Check sheet for the modelled part. Datum: model origin and axes. Units: mm. A direction names the side the tool comes from. Give positions to 0.01 mm unless a question says otherwise; leave off trailing zeros. Write each loop counter-clockwise with the first axis right and the second up, starting at its lowest first coordinate (ties: lowest second). Pieces come first, ordered by that corner, then holes. Notation, with made-up numbers: M 66,-14.5 L 78,-14.5 A20 ccw 78,-6.5 Z; hole C 55,-11.5 d11. An arc over 180 degrees is marked long. Write each question's results on one line, items separated by ' | '. Start each with the question number.
from build123d import *

# Parameters (mm, degrees)
EXTRUDE_1_DEPTH      = 3
CUT_EXTRUDE_2_DEPTH  = 10
CUT_EXTRUDE_6_DEPTH  = 4
SKETCH_12_W          = 293.771267283
SKETCH_12_H          = 20
EXTRUDE_2_DEPTH      = 3
SKETCH_13_R          = 2
CUT_EXTRUDE_9_DEPTH  = 4
CUT_EXTRUDE_10_DEPTH = 10
MM_2_D               = 1.5
CUT_EXTRUDE_11_DEPTH = 4
MM_3_D               = 1.5
FILLET_1_R           = 2
EXTRUDE_3_DEPTH      = 3
SKETCH_4_R           = 1.5
CUT_EXTRUDE_3_DEPTH  = 10


with BuildPart() as part:
    # 草图1 → 凸台-拉伸1 (new body)
    with BuildSketch(Plane.XY):
        Polygon((-31.770103996, 71.767703031), (318.229896004, 71.767703031), (292.931935015, -47.249845949), (-31.770103996, 21.767703031), align=None)
    extrude(amount=EXTRUDE_1_DEPTH)

    # 草图3 → 切除-拉伸2 (cut)
    with BuildSketch(Plane.XY.offset(3)):
        Polygon((-0.469380772, 15.114528924), (0.1543543, 18.048971727), (-31.770103996, 24.834724815), (-31.770103996, 21.767703031), align=None)
        Polygon((176.220922432, -19.375132621), (205.565350454, -25.612483345), (204.941615382, -28.546926147), (175.59718736, -22.309575423), align=None)
    extrude(amount=-CUT_EXTRUDE_2_DEPTH, mode=Mode.SUBTRACT)

    # 草图7 → 切除-拉伸6 (cut, through all)
    with BuildSketch(Plane.XY.offset(3)):
        Polygon((292.931935015, -47.249845949), (239.133816975, -35.814702954), (262.001163287, 71.767703031), (318.229896004, 71.767703031), align=None)
    extrude(amount=-CUT_EXTRUDE_6_DEPTH, mode=Mode.SUBTRACT)

    # 草图12 → 凸台-拉伸2 (add)
    with BuildSketch(Plane.XY.offset(3)):
        with Locations((115.115529646, 81.767703031)):
            Rectangle(SKETCH_12_W, SKETCH_12_H)
    extrude(amount=-EXTRUDE_2_DEPTH)

    # 草图13 → 切除-拉伸9 (cut, through all)
    with BuildSketch(Plane.XY.offset(3)):
        with Locations((-6.770103996, 81.767703031)):
            Circle(SKETCH_13_R)
        with Locations((73.229896004, 81.767703031)):
            Circle(SKETCH_13_R)
        with Locations((153.229896004, 81.767703031)):
            Circle(SKETCH_13_R)
        with Locations((233.229896004, 81.767703031)):
            Circle(SKETCH_13_R)
    extrude(amount=-CUT_EXTRUDE_9_DEPTH, mode=Mode.SUBTRACT)

    # 草图14 → 切除-拉伸10 (cut)
    with BuildSketch(Plane.XY.offset(3)):
        with BuildLine():
            Line((12.482478027, 66.115949401), (209.444028629, 31.386313867))
            ThreePointArc((209.444028629, 31.386313867), (215.933305232, 22.118666422), (206.665657786, 15.629389819))
            Line((206.665657786, 15.629389819), (9.704107184, 50.359025353))
            ThreePointArc((9.704107184, 50.359025353), (3.214830581, 59.626672798), (12.482478027, 66.115949401))
        make_face()
    extrude(amount=-CUT_EXTRUDE_10_DEPTH, mode=Mode.SUBTRACT)

    # 大小mm 暗销槽口2 (through all)
    with Locations(Plane.XY.offset(3)):
        with Locations((0.1543543, 18.048971727), (176.220922432, -19.375132621), (205.565350454, -25.612483345)):
            Hole(MM_2_D / 2)

    # 草图18 → 切除-拉伸11 (cut, through all)
    with BuildSketch(Plane(origin=(0, 0, 0), x_dir=(-1, 0, 0), z_dir=(0, 0, -1))):
        Polygon((-152.291642964, -11.221785469), (-151.667907892, -14.156228271), (-122.32347987, -7.918877547), (-122.947214942, -4.984434744), align=None)
        Polygon((-64.258358898, 7.490266705), (-63.634623826, 4.555823902), (-34.290195804, 10.793174627), (-34.913930876, 13.727617429), align=None)
    extrude(amount=-CUT_EXTRUDE_11_DEPTH, mode=Mode.SUBTRACT)

    # 大小mm 暗销槽口3 (through all)
    with Locations(Plane(origin=(0, 0, 0), x_dir=(-1, 0, 0), z_dir=(0, 0, -1))):
        with Locations((-152.291642964, -11.221785469), (-151.667907892, -14.156228271), (-122.32347987, -7.918877547), (-122.947214942, -4.984434744), (-64.258358898, 7.490266705), (-63.634623826, 4.555823902), (-34.290195804, 10.793174627), (-34.913930876, 13.727617429)):
            Hole(MM_3_D / 2)

    # 圆角1
    fillet_1_edges = [part.edges().sort_by_distance(p)[0] for p in [
        (-31.770103996, 24.834724815, 1.5),
        (239.133816975, -35.814702954, 1.5),
        (262.001163287, 71.767703031, 1.5),
        (-31.770103996, 91.767703031, 1.5),
        (262.001163287, 91.767703031, 1.5),
    ]]
    fillet(fillet_1_edges, radius=FILLET_1_R)

    # 草图21 → 凸台-拉伸3 (add)
    with BuildSketch(Plane.XY.offset(3)):
        Polygon((-91.770103996, 37.588118515), (-13.862424826, 21.028330103), (-13.862424826, 91.767703031), (-81.382896655, 91.767703031), (-91.770103996, 91.767703031), align=None)
    extrude(amount=-EXTRUDE_3_DEPTH)

    # 草图4 → 切除-拉伸3 (cut)
    with BuildSketch(Plane.XY.offset(3)):
        with Locations((-20.141101902, 42.809716012)):
            Circle(SKETCH_4_R)
        with Locations((-0.578149887, 38.651482195)):
            Circle(SKETCH_4_R)
        with Locations((185.269894252, -0.85173906)):
            Circle(SKETCH_4_R)
        with Locations((204.832846267, -5.009972876)):
            Circle(SKETCH_4_R)
    extrude(amount=-CUT_EXTRUDE_3_DEPTH, mode=Mode.SUBTRACT)


solid = part.part
Q1. Release check for a two-part mould opening along Y. For faces 1 (the face through (250.597, 18.114, 1.521)), 2 (the face through (49.39, 10.65, 1.48)), 3 (the face through (122, 29, 3)), 4 (the face through (137.42, -8.06, 1.48)) record: pulls with the +Y half, pulls with the -Y half, needs draft (parallel to the pull), parting line crosses it, or undercut.
Q2. Section check B-B on y = 61.5. Record the boundary of the cut face in (x, z).
Q3. Section check D-D on z = 2.1. State how many separate pieces and enclosed holes the cut face has, plus the area to 3 significant figures.
Q4. Tool access check on faces 5 (the face through (221.29, -32.02, 1.48)), 6 (the face through (190.698, -22.452, 1.521)), 7 (the face through (49.158, 7.633, 1.479)). Record the directions out of +Z, -Z, +X, -X, +Y, -Y that give a thin tool (end or side, any length) a straight path to the whole face; none if there is none.
Q5. Depth check by flat-ended pin: pin 1 Ø2.5 at (x, y) = (-20.14, 42.81) entering from +Z. Enter the tip coordinate at first touch or a pass-through.
Q6. Scan lines: L1, parallel to Y at x = 141, z = 1.35; L2, parallel to Y at x = 141.5, z = 0.35; L3, parallel to X at y = 83.5, z = 0.6. Record each from-to range of solid material in increasing order.
Q7. Section check A-A on x = 53.5. Record the boundary of the cut face in (y, z).
Q8. Section check C-C on x = 213. Record the boundary of the cut face in (y, z), plus the area to 3 significant figures.
Check result:
1) face 1: pulls with the -Y half | face 2: undercut | face 3: needs draft | face 4: undercut
2) outline: M -91.77,0 L 3.79,0 L 3.79,3 L -91.77,3 Z; M 38.66,0 L 259.82,0 L 259.82,3 L 38.66,3 Z
3) separate pieces: 1 | enclosed holes: 11 | area: 28,200 mm^2
4) face 5: +Z, -Z, -X, -Y | face 6: +Z, -Z, -Y | face 7: +Z, -Z
5) pin 1: through
6) L1: -14.96 to -11.89, -8.82 to 27.21, 43.45 to 91.77 | L2: -15.06 to -11.99, -8.93 to 27.12, 43.37 to 91.77 | L3: -91.77 to -7.77, -5.77 to 72.23, 74.23 to 152.23, 154.23 to 232.23, 234.23 to 262
7) outline: M 3.64,0 L 6.71,0 L 6.71,3 L 3.64,3 Z; M 9.78,0 L 42.64,0 L 42.64,3 L 9.78,3 Z; M 58.88,0 L 91.77,0 L 91.77,3 L 58.88,3 Z
8) outline: M -30.26,0 L 17.22,0 L 17.22,3 L -30.26,3 Z; M 29.8,0 L 91.77,0 L 91.77,3 L 29.8,3 Z | area: 328 mm^2
